Here's how the part is built. I have some questions about the finished solid (model axes, mm). Face numbers are marked on the shaded views. A direction names the side the tool comes from. Coordinates: 2 decimals unless noted, no trailing zeros. Order: outer loops, then holes, each group sorted by start corner. A loop starts at its lowest first (then second) coordinate and runs counter-clockwise, first axis right, second up. Notation, with made-up numbers: (-33.75, 34.25) - (13.25, 34.25) arc R26 ccw to (13.25, 53.25) - close; hole circle Ø2 at (-24.5, -29.75). An arc over 180 degrees is marked (long way). Answer as CSV lines item,"result". Start each with the question number.
Q1. For the marked faces 5 and 6, which set-ups out of +Z, -Z, +X, -X, +Y, -Y let a thin tool reach every point of the face, with its end or its side?
Q2. Suppose I cut it at A-A (x = 0). Count the separate pieces of the cut face and the enclosed holes in it, then the cut area to 3 significant figures.
Q3. For pin 1 Ø5.5 at (x, y) = (12, 0.5) entering from +Z; pin 2 Ø8 at (y, z) = (15, 14) entering from +X; pin 3 Ø13 at (x, z) = (12, -99) entering from -Y, each with a flat end and sliding along its axis, tell me the tip position at first contact or that it passes through.
Q4. Suppose I cut it at B-B (z = 0). Please give me the cut outline in (x, y).
Q5. I need wall thicknesses on line 1 (Y direction, x = 4, z = 18.5); line 2 (Z direction, x = 0, y = 2.5); line 3 (Z direction, x = 0, y = -13.8). Which ranges of each line are inside material? Lowest first, please.
Q6. Thinking about a two-plate mould opening in Y: for the marked faces 1, 2, 3 and 4, which applies, released by +Y, released by -Y, zero draft, split by the parting line, or undercut?
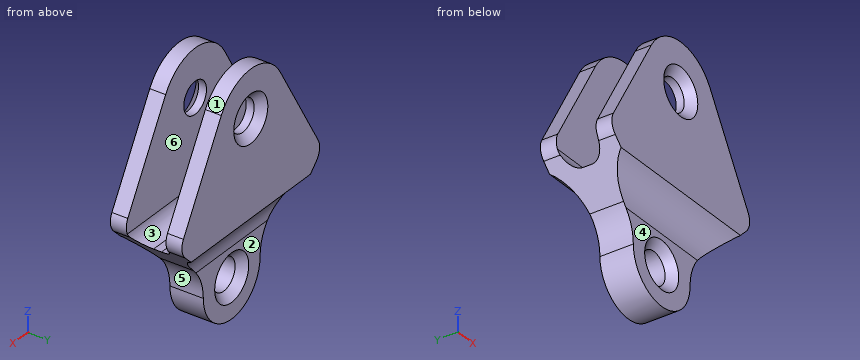
from build123d import *

# Parameters (mm, degrees)
SKETCH1_R               = 10
BOSS_EXTRUDE1_DEPTH     = 22.5
CUT_EXTRUDE1_DEPTH      = 61.66943013
CUT_EXTRUDE1_DEPTH_BACK = 61.66943013
CHAMFER1_SIZE           = 5


with BuildPart() as part:
    # Sketch1 → Boss-Extrude1 (new body, symmetric)
    with BuildSketch(Plane(origin=(0, 0, 0), x_dir=(1, 0, 0), z_dir=(0, 1, 0))):
        with BuildLine():
            Line((-25.980762114, -15), (-59.329684168, 42.762027375))
            ThreePointArc((-59.329684168, 42.762027375), (-60.583878744, 49.067289298), (-57.740497942, 54.833095187))
            Line((-57.740497942, 54.833095187), (-33.786796564, 78.786796564))
            ThreePointArc((-33.786796564, 78.786796564), (-27.283614025, 88.519497029), (-25, 100))
            ThreePointArc((-25, 100), (0, 125), (25, 100))
            ThreePointArc((25, 100), (27.283614025, 88.519497029), (33.786796564, 78.786796564))
            Line((33.786796564, 78.786796564), (57.740497942, 54.833095187))
            ThreePointArc((57.740497942, 54.833095187), (60.583878744, 49.067289298), (59.329684168, 42.762027375))
            Line((59.329684168, 42.762027375), (25.980762114, -15))
            ThreePointArc((25.980762114, -15), (0, -30), (-25.980762114, -15))
        make_face()
        with Locations((0, 100)):
            Circle(SKETCH1_R, mode=Mode.SUBTRACT)
        Circle(SKETCH1_R, mode=Mode.SUBTRACT)
    extrude(amount=BOSS_EXTRUDE1_DEPTH, both=True)

    # Sketch2 → Cut-Extrude1 (cut, two sides)
    with BuildSketch(Plane(origin=(0, 0, 0), x_dir=(0, 0, -1), z_dir=(1, 0, 0))) as cut_extrude1_sk:
        with BuildLine():
            Line((-30, 12.5), (52, 12.5))
            ThreePointArc((52, 12.5), (59.071067812, 9.571067812), (62, 2.5))
            Line((62, 2.5), (62, -2.5))
            ThreePointArc((62, -2.5), (59.071067812, -9.571067812), (52, -12.5))
            Line((52, -12.5), (-30, -12.5))
            Line((-30, -12.5), (-30, 12.5))
        make_face()
        with BuildLine():
            Line((81.354156504, 10.5), (125, 10.5))
            Line((125, 10.5), (125, 22.5))
            Line((125, 22.5), (78.786796564, 22.5))
            Line((78.786796564, 22.5), (60, 22.5))
            ThreePointArc((60, 22.5), (69.10670779, 13.705505282), (81.354156504, 10.5))
        make_face()
        with BuildLine():
            Line((125, -22.5), (125, -10.5))
            Line((125, -10.5), (81.354156504, -10.5))
            ThreePointArc((81.354156504, -10.5), (69.10670779, -13.705505282), (60, -22.5))
            Line((60, -22.5), (78.786796564, -22.5))
            Line((78.786796564, -22.5), (125, -22.5))
        make_face()
    extrude(amount=CUT_EXTRUDE1_DEPTH, mode=Mode.SUBTRACT)
    extrude(cut_extrude1_sk.sketch, amount=-CUT_EXTRUDE1_DEPTH_BACK, mode=Mode.SUBTRACT)

    # Chamfer1
    chamfer1_edges = [part.edges().sort_by_distance(p)[0] for p in [
        (-10, -22.5, 0),
        (-10, 22.5, 0),
        (-10, -10.5, -100),
        (-10, 10.5, -100),
    ]]
    chamfer(chamfer1_edges, length=CHAMFER1_SIZE)


solid = part.part
Here are the results:
1,face 5,"-Z, +X, +Y, -Y"
1,face 6,"+Z, +X, -X"
2,separate pieces,"4"
2,enclosed holes,"0"
2,area,"2,390 mm²"
3,pin 1,"stops at z = -61.97"
3,pin 2,"stops at x = 28.87"
3,pin 3,"stops at y = -10.5"
4,outline,"(-34.64, -22.5) - (-15, -22.5) - (-10, -17.5) - (-10, -12.5) - (-34.64, -12.5) - close; (-34.64, 12.5) - (-10, 12.5) - (-10, 17.5) - (-15, 22.5) - (-34.64, 22.5) - close; (10, -17.5) - (15, -22.5) - (34.64, -22.5) - (34.64, -12.5) - (10, -12.5) - close; (10, 12.5) - (34.64, 12.5) - (34.64, 22.5) - (15, 22.5) - (10, 17.5) - close"
5,line 1,"y = -22.5 to -12.5, 12.5 to 22.5"
5,line 2,"z = -125 to -110, -90 to -62"
5,line 3,"z = -68.94 to -10, 10 to 30"
6,face 1,"zero draft"
6,face 2,"released by +Y"
6,face 3,"undercut"
6,face 4,"released by -Y"
